```python
from build123d import *

# Parameters (mm, degrees)
SKETCH10_R         = 1.833087105
CUT_EXTRUDE2_DEPTH = 1.6129
CUT_EXTRUDE2_DRAFT = -45
CUT_EXTRUDE1_DEPTH = 1.6129


with BuildPart() as part:
    # Sketch2 → Revolve1 (revolve)
    with BuildSketch(Plane(origin=(0, 0, 0), x_dir=(0, 0, -1), z_dir=(1, 0, 0))):
        with BuildLine():
            Line((-7.872984, 5.2197), (-4.7117, 2.471637744))
            ThreePointArc((-4.7117, 2.471637744), (-4.63858483, 2.428138789), (-4.554866229, 2.413))
            Line((-4.554866229, 2.413), (7.3421875, 2.413))
            Line((7.3421875, 2.413), (7.9375, 1.8176875))
            Line((7.9375, 1.8176875), (7.9375, 0))
            Line((7.9375, 0), (-7.9375, 0))
            Line((-7.9375, 0), (-7.9375, 5.2197))
            Line((-7.9375, 5.2197), (-7.872984, 5.2197))
        make_face()
    revolve(axis=Axis((0, 0, -7.9375), (0, 0, 1)))


with BuildPart() as cut_extrude2_tool:
    # Sketch10 → Cut-Extrude2 (with draft: the straight prism first)
    with BuildSketch(Plane.XY.offset(7.9375)):
        Circle(SKETCH10_R)
    extrude(amount=-CUT_EXTRUDE2_DEPTH)
    # Cut-Extrude2: the draft: its side faces are tilted about the plane it starts from
    cut_extrude2_sides = [cut_extrude2_tool.faces().sort_by_distance(p)[0] for p in [
        (-1.833087105, 0, 7.13105),
    ]]
    draft(cut_extrude2_sides, Plane.XY.offset(7.9375), CUT_EXTRUDE2_DRAFT)


with BuildPart() as part_1:
    add(part.part)

    # Cut-Extrude2: cut by cut_extrude2_tool
    add(cut_extrude2_tool.part, mode=Mode.SUBTRACT)

    # Sketch9 → Cut-Extrude1 (cut)
    with BuildSketch(Plane.XY.offset(7.9375)):
        Polygon((1.5875, -0.916543552), (1.5875, 0.916543552), (0, 1.833087105), (-1.5875, 0.916543552), (-1.5875, -0.916543552), (0, -1.833087105), align=None)
    extrude(amount=-CUT_EXTRUDE1_DEPTH, mode=Mode.SUBTRACT)


solid = part_1.part
```
Input: part model. Units: mm. Frame: model coordinates. A direction names the side the tool comes from. Coordinates: 2 decimals unless noted, no trailing zeros. Write each loop counter-clockwise with the first axis right and the second up, starting at its lowest first coordinate (ties: lowest second). Pieces come first, ordered by that corner, then holes.
1) Section A-A on y = 0. Output: boundary loops of the cut face in (x, z).
2) Mould query, pull axis Y, two halves, no side actions, for faces 3 (the cylindrical face through (1.468, -1.915, -1.477)), 4 (the flat face through (2, 0, 7.938)), 5 (the flat face through (0.8, 1.37, 7.14)). Classes: pulls with the +Y half, pulls with the -Y half, needs draft (parallel to the pull), parting line crosses it, or undercut.
3) Section B-B on z = 1. Output: boundary loops of the cut face in (x, y).
4) Material intervals for line 1 along Y through (x, z) = (0.5, 7.25); line 2 along Y through (x, z) = (-0.75, 2.5); line 3 along Y through (x, z) = (-1.5, -2.25), sorted ascending.
5) Pin query (flat end, axial travel): pin 1 Ø6 at (x, y) = (1, 3.5) entering from -Z; pin 2 Ø6 at (y, z) = (0, -3.5) entering from -X; pin 3 Ø4 at (x, z) = (-1.5, -5.5) entering from -Y; pin 4 Ø1.6 at (x, y) = (0.5, -0.5) entering from +Z. Return the tip coordinate at first contact, or that it passes through.
6) Set-up query: faces 1 (the flat face through (-0.783, 1.381, 7.142)), 2 (the conical face through (1.59, -2.07, 4.87)). Return all of +Z, -Z, +X, -X, +Y, -Y with unobstructed straight access to the full face (end or side cutting, diameter ignored); none if empty.
Check result:
1. outline: (-5.22, 7.87) - (-2.47, 4.71) arc R0.24 cw to (-2.41, 4.55) - (-2.41, -7.34) - (-1.82, -7.94) - (1.82, -7.94) - (2.41, -7.34) - (2.41, 4.55) arc R0.24 cw to (2.47, 4.71) - (5.22, 7.87) - (5.22, 7.94) - (1.83, 7.94) - (1.59, 7.69) - (1.59, 6.32) - (-1.59, 6.32) - (-1.59, 7.69) - (-1.83, 7.94) - (-5.22, 7.94) - close
2. face 3: parting line crosses it
2. face 4: needs draft
2. face 5: undercut
3. outline: circle Ø4.83 at (0, 0)
4. line 1: y = -4.65 to -1.54, 1.54 to 4.65
4. line 2: y = -2.29 to 2.29
4. line 3: y = -1.89 to 1.89
5. pin 1: stops at z = -7.94
5. pin 2: stops at x = -2.41
5. pin 3: stops at y = -2.41
5. pin 4: stops at z = 6.32
6. face 1: +Z
6. face 2: -Z
